Job drawing, mm, ordinate dimensions from the low corner. One solid piece. Coordinates: 2 decimals unless noted, no trailing zeros. Loops run counter-clockwise (first coordinate to the right, second up) from the corner with the lowest first, then second, coordinate; pieces in that order, holes last. Notation, with made-up numbers: (-35, -26) - (12, -26) arc R31 cw to (12, 13) - close; hole circle Ø5 at (53.25, 39.25). An arc over 180 degrees is marked (long way). One line per question, with ' | ' between items. Start each with the question number.
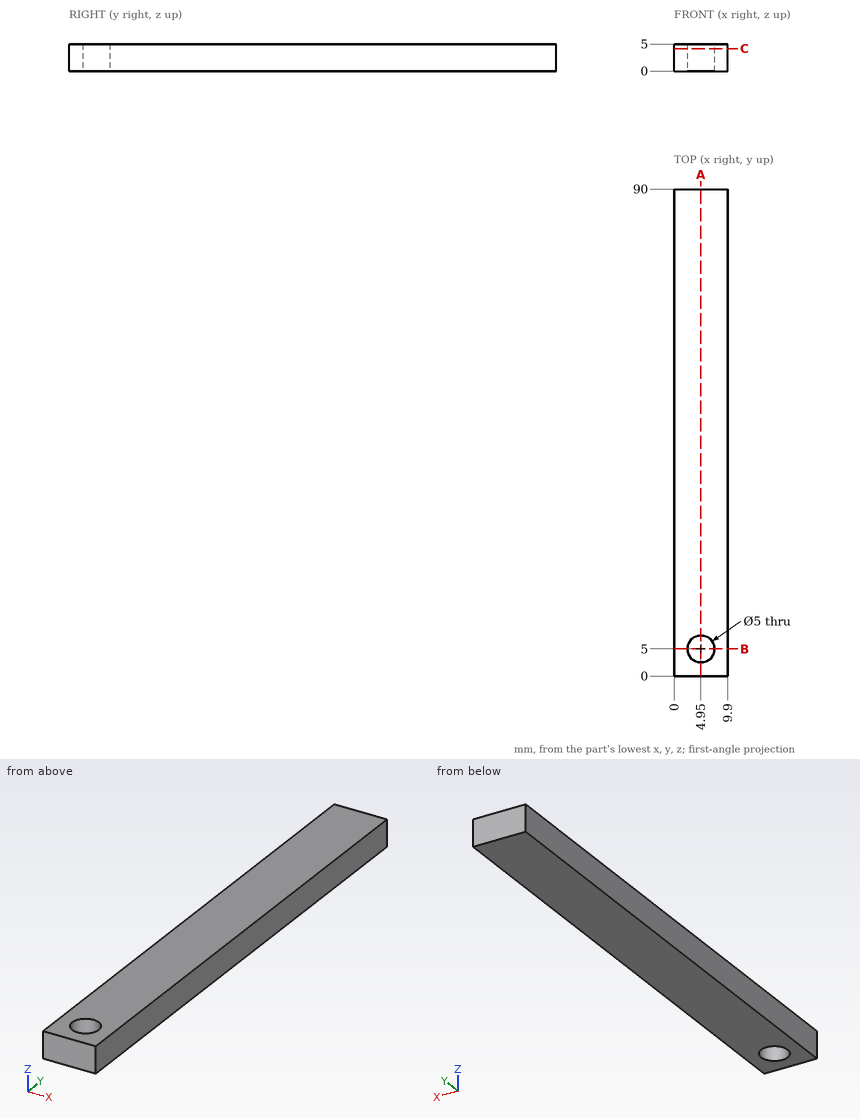
1) Band-saw the part on C-C on z = 4.15. List the corners of the cut face in (x, y).
2) Wall check: line 1 along X through (y, z) = (5, 1.2); line 2 along Y through (x, z) = (4.95, 3.1); line 3 along X through (y, z) = (6.5, 3.8). Give the ranges that are in metal, low to high. Write a range as [from, to].
3) Band-saw the part on A-A on x = 4.95. List the corners of the cut face in (y, z).
4) Band-saw the part on B-B on y = 5. List the corners of the cut face in (x, z), then the cut area to 3 significant figures.
Values found:
1) outline: (0, 0) - (9.9, 0) - (9.9, 90) - (0, 90) - close; hole circle Ø5 at (4.95, 5)
2) line 1: [0, 2.45], [7.45, 9.9] | line 2: [0, 2.5], [7.5, 90] | line 3: [0, 2.95], [6.95, 9.9]
3) outline: (0, 0) - (2.5, 0) - (2.5, 5) - (0, 5) - close; (7.5, 0) - (90, 0) - (90, 5) - (7.5, 5) - close
4) outline: (0, 0) - (2.45, 0) - (2.45, 5) - (0, 5) - close; (7.45, 0) - (9.9, 0) - (9.9, 5) - (7.45, 5) - close | area: 24.5 mm²
